The listing builds one solid part. Answer for the finished solid, in the listing's coordinates (mm). Round coordinates to 2 decimals unless told otherwise and drop trailing zeros. Write each loop counter-clockwise with the first axis right and the second up, starting at its lowest first coordinate (ties: lowest second). Pieces come first, ordered by that corner, then holes. Notation, with made-up numbers: (64, 3) - (109, 3) arc R15 cw to (109, 30) - close; hole circle Ø10 at (-34.5, -40). An arc over 180 degrees is marked (long way). Answer in a Markdown table with one row per item.
from build123d import *

# Parameters (mm, degrees)
BOSS_EXTRUDE1_DEPTH = 3
CIRPATTERN1_COUNT   = 4
CUT_EXTRUDE1_REACH  = 5


with BuildPart() as part:
    # Sketch1 → Boss-Extrude1 (new body)
    with BuildSketch(Plane.XY):
        Polygon((3.5, 26), (1.5, 24), (1.5, 21), (0, 21), (0, 18), (1.5, 18), (1.5, 15), (0, 15), (0, 12), (0, 9), (0, 6), (0, 3), (0, 0), (3, 0), (6, 0), (9, 0), (12, 0), (15, 0), (15, 1.5), (18, 1.5), (18, 0), (21, 0), (21, 1.5), (24, 1.5), (26, 3.5), (26, 26), align=None)
    boss_extrude1 = extrude(amount=BOSS_EXTRUDE1_DEPTH)

    # CirPattern1: Boss-Extrude1 ×4 about axis
    cirpattern1_axis = Axis((0, 0, 0), (0, 0, 1))
    for i in range(1, CIRPATTERN1_COUNT):
        add(boss_extrude1.rotate(cirpattern1_axis, i * 360 / CIRPATTERN1_COUNT))

    # Sketch2 → Cut-Extrude1 (cut, up to next)
    with BuildSketch(Plane.XY, mode=Mode.PRIVATE) as cut_extrude1_sk1:
        with BuildLine():
            Line((26, 26), (36, 26))
            Line((36, 26), (36, -26))
            Line((36, -26), (26, -26))
            ThreePointArc((26, -26), (22.568883707, -11.465558146), (13, 0))
            ThreePointArc((13, 0), (22.568883707, 11.465558146), (26, 26))
        make_face()
    cut_extrude1_tool1 = extrude(cut_extrude1_sk1.sketch, amount=CUT_EXTRUDE1_REACH, mode=Mode.PRIVATE) & part.part
    add(cut_extrude1_tool1.solids().sort_by_distance((28.547836, 0, 0))[0], mode=Mode.SUBTRACT)


solid = part.part
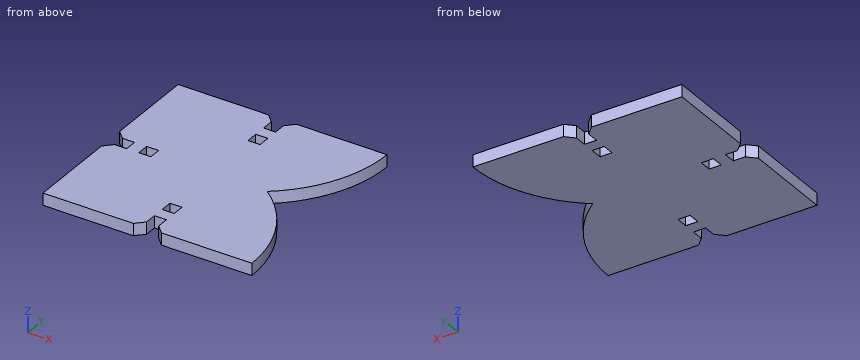
(1) Section B-B (y = -22) is taken. Give the vertices of the cut face in (x, z), and give its area (3 significant figures).
Checked values:
| item | result |
|---|---|
| outline | (-26, 0) - (-1.5, 0) - (-1.5, 3) - (-26, 3) - close; (1.5, 0) - (25.75, 0) - (25.75, 3) - (1.5, 3) - close |
| area | 146 mm2 |
(2) Find the intervals of material crossed by line 1 (Y direction, x = -22, z = 2.1); line 2 (X direction, y = -22, z = 0.6); line 3 (Y direction, x = 17, z = 2.2), in increasing order.
Checked values:
| item | result |
|---|---|
| line 1 | y = -26 to -1.5, 1.5 to 26 |
| line 2 | x = -26 to -1.5, 1.5 to 25.75 |
| line 3 | y = -26 to -3.55, 3.55 to 26 |
(3) Section D-D (y = 8.5) is taken. Give the vertices of the cut face in (x, z), and give its area (3 significant figures).
Checked values:
| item | result |
|---|---|
| outline | (-26, 0) - (20.89, 0) - (20.89, 3) - (-26, 3) - close |
| area | 141 mm2 |
(4) Section C-C (z = 1.95) is taken. State how many separate pieces and enclosed holes the cut face has, and give its area (3 significant figures).
Checked values:
| item | result |
|---|---|
| separate pieces | 1 |
| enclosed holes | 3 |
| area | 2,420 mm2 |
(5) Section A-A (x = -22.5) is taken. Give the vertices of the cut face in (y, z), and give its area (3 significant figures).
Checked values:
| item | result |
|---|---|
| outline | (-26, 0) - (-1.5, 0) - (-1.5, 3) - (-26, 3) - close; (1.5, 0) - (26, 0) - (26, 3) - (1.5, 3) - close |
| area | 147 mm2 |
(6) Flat-ended cylindrical pins translate along their axes: pin 1 (1.5 mm diameter, centred on x = -0.5, z = 2, fed in from -Y); pin 2 (1.5 mm diameter, centred on y = -0.5, z = 2, fed in from +X). Find the tip coordinate at first contact, or state that the pin passes through.
Checked values:
| item | result |
|---|---|
| pin 1 | stops at y = -21 |
| pin 2 | stops at x = 14.56 |
